Here's how the part is built. I have some questions about the finished solid (model axes, mm). A direction names the side the tool comes from. Coordinates: 2 decimals unless noted, no trailing zeros. Write each loop counter-clockwise with the first axis right and the second up, starting at its lowest first coordinate (ties: lowest second). Pieces come first, ordered by that corner, then holes.
Item 1: I want a section at B-B (x = 0). Please give me the cut outline in (y, z).
Item 2: If we mould it in two halves opening along Y, with no side actions, what happens to faces 1 (the face through (23.372, -7.717, -0.11)), 2 (the face through (-18, 0, -10)), 3 (the face through (-18, -10, -10))? For each: pulls with the +Y half, pulls with the -Y half, needs draft (parallel to the pull), parting line crosses it, or undercut.
Item 3: I'm going to push flat-ended pins straight in: P1, Ø2, axis at x = -7.5, y = -3, coming from the +Z side; P2, Ø1, axis at y = -5.5, z = 4.5, coming from the +X side; P3, Ø4.5, axis at y = -4.67, z = 0, coming from the -X side. Where does each tip first touch, or does it pass through?
Item 4: I want a section at A-A (z = 0). Please give me the cut outline in (x, y), and give its area (3 significant figures).
Item 5: Please list where these lines run through material, in increasing order: line 1 (Z direction, x = 0, y = -5.25); line 2 (Z direction, x = 13, y = -3.75); line 3 (X direction, y = -1.5, z = -1.5).
Item 6: I want a section at D-D (y = -1.25). Please give me the cut outline in (x, z).
Item 7: For faces 4 (the face through (-23.372, -7.164, 0.11)), 5 (the face through (25.754, -4.93, 8.11)), which set-ups out of +Z, -Z, +X, -X, +Y, -Y let a thin tool reach every point of the face, with its end or its side?
Item 8: I want a section at C-C (y = -5.75). Please give me the cut outline in (x, z).
from build123d import *

# Parameters (mm, degrees)
F0_R     = 27.0011142562
F0_R_2   = 20
F1_DEPTH = 10
F3_D     = 5
F3_DEPTH = 27.0021142562
F5_D     = 5
F5_DEPTH = 27.0021143562


with BuildPart() as f1:
    # F0 (on Front) → F1 (new body)
    with BuildSketch(Plane.XZ):
        Circle(F0_R)
        Circle(F0_R_2, mode=Mode.SUBTRACT)
    extrude(amount=F1_DEPTH)

    # F3 (through all, one way)
    with BuildSketch(Plane.YZ):
        with Locations((-4.6664830297, 0)):
            Circle(F3_D / 2)
    extrude(amount=-F3_DEPTH, mode=Mode.SUBTRACT)

    # F5 (through all, one way)
    with BuildSketch(Plane(origin=(0, 0, 0), x_dir=(0, 1, 0), z_dir=(-1, 0, 0))):
        with Locations((-5.219371058, 0)):
            Circle(F5_D / 2)
    extrude(amount=-F5_DEPTH, mode=Mode.SUBTRACT)


solid = f1.part
Answer:
1. outline: (-10, -27) - (0, -27) - (0, -20) - (-10, -20) - close; (-10, 20) - (0, 20) - (0, 27) - (-10, 27) - close
2. face 1: undercut
2. face 2: pulls with the +Y half
2. face 3: pulls with the -Y half
3. P1: stops at z = 26.21
3. P2: stops at x = 26.7
3. P3: stops at x = 19.89
4. outline: (-27, -10) - (-20, -10) - (-20, -7.17) - (-27, -7.17) - close; (-27, -2.17) - (-20, -2.17) - (-20, 0) - (-27, 0) - close; (20, -10) - (27, -10) - (27, -7.72) - (20, -7.72) - close; (20, -2.72) - (27, -2.72) - (27, 0) - (20, 0) - close
4. area: 70.0 mm2
5. line 1: z = -27 to -20, 20 to 27
5. line 2: z = -23.67 to -15.2, 15.2 to 23.67
5. line 3: x = -26.96 to -19.94, 19.94 to 26.96
6. outline: circle Ø54 at (0, 0); hole circle Ø40 at (0, 0)
7. face 4: -X
7. face 5: +Y, -Y
8. outline: (-26.91, -2.25) arc R27 ccw to (26.89, -2.44) - (19.85, -2.44) arc R20 cw to (-19.87, -2.25) - close; (-26.91, 2.25) - (-19.87, 2.25) arc R20 cw to (19.85, 2.44) - (26.89, 2.44) arc R27 ccw to start
